from build123d import *

# Parameters (mm, degrees)
SKETCH1_W           = 21.5
SKETCH1_H           = 5.5
BOSS_EXTRUDE1_DEPTH = 8
SKETCH2_R           = 1.75
CUT_EXTRUDE1_DEPTH  = 6.5
CUT_EXTRUDE2_DEPTH  = 2.5
BOSS_EXTRUDE3_DEPTH = 1
BOSS_EXTRUDE4_DEPTH = 1
FILLET1_R           = 2


with BuildPart() as part:
    # Sketch1 → Boss-Extrude1 (new body)
    with BuildSketch(Plane.XY):
        with Locations((10.75, -2.75)):
            Rectangle(SKETCH1_W, SKETCH1_H)
    extrude(amount=BOSS_EXTRUDE1_DEPTH)

    # Sketch2 → Cut-Extrude1 (cut, through all)
    with BuildSketch(Plane.XZ.offset(5.5)):
        with Locations((3.875, 4)):
            Circle(SKETCH2_R)
        with Locations((17.625, 4)):
            Circle(SKETCH2_R)
    extrude(amount=-CUT_EXTRUDE1_DEPTH, mode=Mode.SUBTRACT)

    # Sketch3 → Cut-Extrude2 (cut)
    with BuildSketch(Plane(origin=(0, 0, 0), x_dir=(1, 0, 0), z_dir=(0, 1, 0))):
        Polygon((6.875, -5.732050808), (6.875, -2.267949192), (3.875, -0.535898385), (0.875, -2.267949192), (0.875, -5.732050808), (3.875, -7.464101615), align=None)
        Polygon((20.625, -2.267949192), (17.625, -0.535898385), (14.625, -2.267949192), (14.625, -5.732050808), (17.625, -7.464101615), (20.625, -5.732050808), align=None)
    extrude(amount=-CUT_EXTRUDE2_DEPTH, mode=Mode.SUBTRACT)

    # Sketch4 → Boss-Extrude3 (add)
    with BuildSketch(Plane.XY.offset(1)):
        Polygon((7.5, -5.5), (14, -5.5), (12.5, -6.5), (9, -6.5), align=None)
    extrude(amount=BOSS_EXTRUDE3_DEPTH)

    # Sketch5 → Boss-Extrude4 (add)
    with BuildSketch(Plane.XY.offset(7)):
        Polygon((7.5, -5.5), (9, -6.5), (12.5, -6.5), (14, -5.5), align=None)
    extrude(amount=-BOSS_EXTRUDE4_DEPTH)

    # Fillet1
    fillet1_edges = [part.edges().sort_by_distance(p)[0] for p in [
        (21.5, -2.75, 8),
        (21.5, -2.75, 0),
        (0, -2.75, 0),
        (0, -2.75, 8),
    ]]
    fillet(fillet1_edges, radius=FILLET1_R)


solid = part.part
Geometry check sheet. Reference: the model listing, model coordinates, mm. A direction names the side the tool comes from. Give positions to 0.01 mm unless a question says otherwise; leave off trailing zeros. Loops run counter-clockwise (first coordinate to the right, second up) from the corner with the lowest first, then second, coordinate; pieces in that order, holes last.
(1) Depth check by flat-ended pin: pin 1 Ø1 at (y, z) = (-4.5, 7) entering from +X; pin 2 Ø4 at (x, z) = (3.875, 4) entering from +Y; pin 3 Ø0.8 at (x, y) = (10, -6) entering from +Z. Enter the tip coordinate at first touch or a pass-through.
From the geometry:
pin 1: stops at x = 21.44
pin 2: stops at y = -2.5
pin 3: stops at z = 7
(2) Release check for a two-part mould opening along X. For faces 1 (the flat face through (11, -6, 7)), 2 (the flat face through (8.26, -6.007, 1.493)), 3 (the flat face through (2, -2.5, 5)), 4 (the flat face through (13.24, -6.007, 6.507)) record: released by +X, released by -X, zero draft, split by the parting line, or undercut.
From the geometry:
face 1: zero draft
face 2: released by -X
face 3: undercut
face 4: released by +X
(3) Thickness scan on L1, parallel to X at y = -1.75, z = 5 (3 decimals); L2, parallel to X at y = -2, z = 7.25; L3, parallel to Z at x = 18.25, y = -0.75. Record the ranges inside material, lowest first.
From the geometry:
L1: x = 0 to 0.875, 6.875 to 14.625, 20.625 to 21.5
L2: x = 0.44 to 3.5, 4.25 to 17.25, 18 to 21.06
L3: z = 0 to 0.9, 7.1 to 8
(4) Set-up check for faces 5 (the flat face through (11, -3, 0)), 6 (the flat face through (2.354, -1.232, 6.586)): record each of +Z, -Z, +X, -X, +Y, -Y from which the full face is reachable in a straight line by a thin tool's end or side.
From the geometry:
face 5: -Z, +X, -X, +Y, -Y
face 6: +Y
(5) Section check D-D on x = 9.5. Record the cut outline in (y, z), then the cut area to 3 significant figures.
From the geometry:
outline: (-6.5, 1) - (-5.5, 1) - (-5.5, 0) - (0, 0) - (0, 8) - (-5.5, 8) - (-5.5, 7) - (-6.5, 7) - (-6.5, 6) - (-5.5, 6) - (-5.5, 2) - (-6.5, 2) - close
area: 46.0 mm2
(6) Section check B-B on x = 5. Record the cut outline in (y, z), then the cut area to 3 significant figures.
From the geometry:
outline: (-5.5, 0) - (0, 0) - (0, 1.19) - (-2.5, 1.19) - (-2.5, 2.66) - (-5.5, 2.66) - close; (-5.5, 5.34) - (-2.5, 5.34) - (-2.5, 6.81) - (0, 6.81) - (0, 8) - (-5.5, 8) - close
area: 21.9 mm2
(7) Section check C-C on z = 5.25. Record the cut outline in (x, y) (3 decimals), then the cut area to 3 significant figures.
From the geometry:
outline: (0, -5.5) - (2.65, -5.5) - (2.65, -2.5) - (0.875, -2.5) - (0.875, 0) - (0, 0) - close; (5.1, -5.5) - (16.4, -5.5) - (16.4, -2.5) - (14.625, -2.5) - (14.625, 0) - (6.875, 0) - (6.875, -2.5) - (5.1, -2.5) - close; (18.85, -5.5) - (21.5, -5.5) - (21.5, 0) - (20.625, 0) - (20.625, -2.5) - (18.85, -2.5) - close
area: 73.6 mm2
(8) Section check A-A on y = -1.75. Record the cut outline in (x, z) (3 decimals).
From the geometry:
outline: (0, 2) arc R2 ccw to (2, 0) - (19.5, 0) arc R2 ccw to (21.5, 2) - (21.5, 6) arc R2 ccw to (19.5, 8) - (2, 8) arc R2 ccw to (0, 6) - close; hole (0.875, 2.268) - (3.875, 0.536) - (6.875, 2.268) - (6.875, 5.732) - (3.875, 7.464) - (0.875, 5.732) - close; hole (14.625, 2.268) - (17.625, 0.536) - (20.625, 2.268) - (20.625, 5.732) - (17.625, 7.464) - (14.625, 5.732) - close
